Read the model definition and answer for the solid it produces. Units are mm, in the model's axes. Coordinates: 2 decimals unless noted, no trailing zeros. Loops run counter-clockwise (first coordinate to the right, second up) from the corner with the lowest first, then second, coordinate; pieces in that order, holes last.
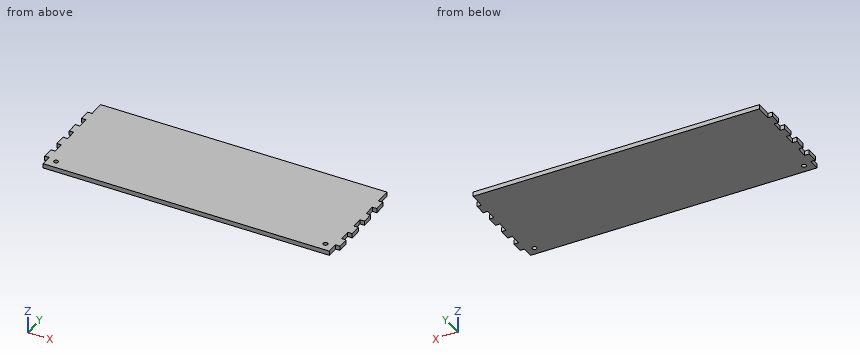
Autodesk Inventor part; units mm, degrees
ref_plane "YZ Plane" through (0, 0, 0) normal (1, 0, 0) x (0, 1, 0)
ref_plane "XZ Plane" through (0, 0, 0) normal (0, 1, 0) x (-1, 0, 0)
ref_plane "XY Plane" through (0, 0, 0) normal (0, 0, 1) x (1, 0, 0)
sketch "Эскиз1" plane through (0, 0, 0) normal (0, 0, 1) x (1, 0, 0)
  line L0 (-26.3955, 0) -> (-26.3955, 30)
  line L1 (228.6045, 0) -> (228.6045, 30)
  circle A0 centre (221.1045, 7.5) radius 2
  circle A1 centre (-18.8955, 7.5) radius 2
  line L2 (-26.3955, 60.0004) -> (-30.3955, 60.0004)
  line L3 (-26.3955, 60.0004) -> (228.6045, 60.0004)
  line L4 (228.6045, 60.0004) -> (228.6045, 0)
  line L5 (228.6045, 0) -> (-26.3955, 0)
  line L6 (-26.3955, 0) -> (-26.3955, 60.0004)
  point P0 (0, 0)
  dimension "d34" = 7.5
  dimension "d35" = 7.5
  dimension "d36" = 255
extrude "Выдавливание1" add sketch "Эскиз1" along normal blind 4
thicken "Толщина1" operation add thickness 4 both sides no extend neighbours yes toward (1, 0, 0) faces at (228.6045, 10, 1.3333)
thicken "Толщина2" operation add thickness 4 both sides no extend neighbours yes toward (-1, 0, 0) faces at (-26.3955, 40.0003, 2.6667)
sketch "Эскиз2" plane through (0, 0, 4) normal (0, 0, 1) x (1, 0, 0)
  line L0 (232.6045, 60.0004) -> (-30.3955, 60.0004)
  line L1 (-30.3955, 60.0004) -> (232.6045, 60.0004)
  line L2 (232.6045, 60.0004) -> (232.6045, 90.0004)
  line L3 (232.6045, 90.0004) -> (-30.3955, 90.0004)
  line L4 (-30.3955, 90.0004) -> (-30.3955, 60.0004)
  point P0 (0, 0)
  dimension "d6" = 30
  dimension "d37" = 263
extrude "Выдавливание2" add sketch "Эскиз2" against normal blind 4
sketch "Эскиз3" plane through (0, 0, 4) normal (0, 0, 1) x (1, 0, 0)
  line L0 (-30.3955, 90.0004) -> (-30.3955, 0)
  line L1 (-30.3955, 90.0004) -> (-26.3955, 90.0004)
  line L2 (-26.3955, 90.0004) -> (-26.3955, 80.0004)
  line L3 (-26.3955, 80.0004) -> (-30.3955, 80.0004)
  line L4 (-30.3955, 80.0004) -> (-30.3955, 90.0004)
  point P0 (0, 0)
  dimension "d9" = 4
  dimension "d10" = 10
extrude "Выдавливание3" cut sketch "Эскиз3" against normal blind 4
pattern_linear "Прямоуг.массив1" count 5 spacing 20 along (0, -1, 0) of "Выдавливание3"
thicken "Толщина3" operation add thickness 1 both sides no extend neighbours yes toward (1, 0, 0) faces at (-30.3955, 0.0003, 1.3333) (-29.0622, 0.0004, 2.6667)
sketch "Эскиз4" plane through (0, 0, 4) normal (0, 0, 1) x (1, 0, 0)
  line L0 (232.6045, 90.0004) -> (228.6045, 90.0004)
  line L1 (228.6045, 90.0004) -> (228.6045, 80.0004)
  line L2 (228.6045, 80.0004) -> (232.6045, 80.0004)
  line L3 (232.6045, 80.0004) -> (232.6045, 90.0004)
  point P0 (0, 0)
  dimension "d18" = 4
  dimension "d19" = 10
extrude "Выдавливание4" cut sketch "Эскиз4" against normal blind 4
pattern_linear "Прямоуг.массив2" count 5 spacing 20 along (0, -1, 0) of "Выдавливание4"
thicken "Толщина4" operation add thickness 1 both sides no extend neighbours yes toward (-1, 0, 0) faces at (232.6045, 0.0001, 1.3333) (229.9378, 0.0004, 2.6667)
sketch "Эскиз5" plane through (0, 0, 4) normal (0, 0, 1) x (1, 0, 0)
  line L0 (-26.3955, 90.0004) -> (228.6045, 90.0004)
  line L1 (-26.3955, 90.0004) -> (-21.3955, 90.0004)
  line L2 (-21.3955, 90.0004) -> (-21.3955, 94.0004)
  line L3 (-21.3955, 94.0004) -> (-26.3955, 94.0004)
  line L4 (-26.3955, 94.0004) -> (-26.3955, 90.0004)
  point P0 (0, 0)
  dimension "d27" = 5
  dimension "d28" = 4
extrude "Выдавливание5" add sketch "Эскиз5" against normal blind 4
pattern_linear "Прямоуг.массив3" count 51 spacing 5 along (1, 0, 0) of "Выдавливание5"
properties part number "KB33-046-004-014 - Лицевая вертикальня пластина" material "Пластик АБС"
Item 1: Given pin 1 (2 mm diameter, centred on y = 67.5, z = 2, fed in from +X); pin 2 (1.2 mm diameter, centred on x = 230, z = 1.5, fed in from -Y); pin 3 (2 mm diameter, centred on x = -28.5, z = 2, fed in from +Y), each flat-ended and moving along its own axis, determine where each tip first touches the part or whether it passes through.
Numbers:
pin 1: stops at x = 228.6
pin 2: stops at y = 10
pin 3: stops at y = 80
Item 2: Find the intervals of material crossed by line 1 along X through (y, z) = (7.5, 2.3); line 2 along X through (y, z) = (6.5, 3.15); line 3 along X through (y, z) = (41, 1.55), in increasing order.
Numbers:
line 1: x = -26.4 to -20.9, -16.9 to 219.1, 223.1 to 228.6
line 2: x = -26.4 to -20.63, -17.16 to 219.37, 222.84 to 228.6
line 3: x = -26.4 to 228.6
Item 3: A cutting plane is placed at A-A on z = 3.05. Give the number of separate pieces and of enclosed holes in the cut face, then the cut area to 3 significant figures.
Numbers:
separate pieces: 1
enclosed holes: 2
area: 24,300 mm2
Item 4: A cutting plane is placed at B-B on y = 26. Determine the outline of the cut face in (x, z).
Numbers:
outline: (-26.4, 0) - (228.6, 0) - (228.6, 4) - (-26.4, 4) - close
